Check sheet for the drawn part. Datum: minimum x, y, z corner. Units: mm. A direction names the side the tool comes from. Round coordinates to 2 decimals unless told otherwise and drop trailing zeros. Write each loop counter-clockwise with the first axis right and the second up, starting at its lowest first coordinate (ties: lowest second). Pieces come first, ordered by that corner, then holes. Notation, with made-up numbers: M 55.25,39 L 110.25,39 A30 ccw 110.25,77 Z; hole C 36.5,-23 d4. An arc over 180 degrees is marked long. Put each result on its own line as item: value.
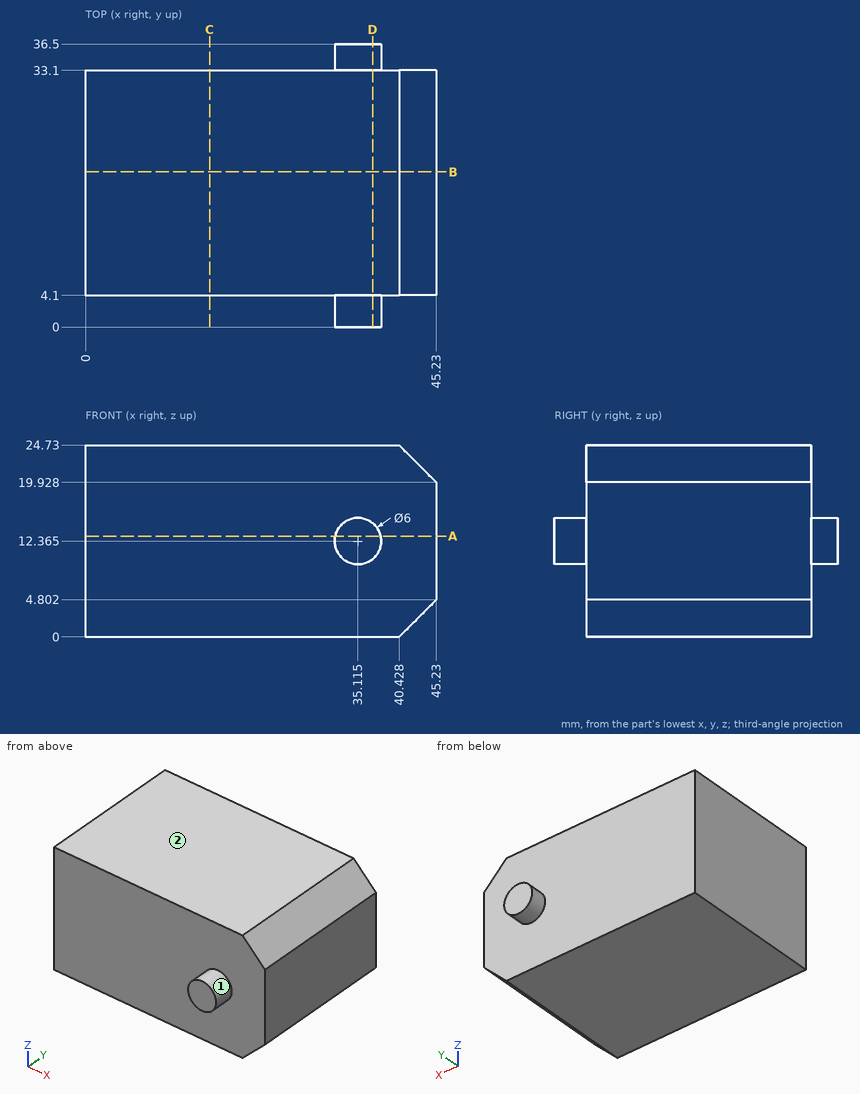
1. Depth check by flat-ended pin: pin 1 Ø1 at (y, z) = (28, 2.5) entering from +X; pin 2 Ø3 at (x, z) = (26.5, 2.5) entering from +Y. Enter the tip coordinate at first touch or a pass-through.
Computed values:
pin 1: stops at x = 43.43
pin 2: stops at y = 33.1
2. Cross-section at D-D (x = 37). Enter the section's corners in (y, z), then the cut area to 3 significant figures.
Computed values:
outline: M 0,10.03 L 4.1,10.03 L 4.1,0 L 33.1,0 L 33.1,10.03 L 36.5,10.03 L 36.5,14.7 L 33.1,14.7 L 33.1,24.73 L 4.1,24.73 L 4.1,14.7 L 0,14.7 Z
area: 752 mm2
3. Cross-section at A-A (z = 13). Enter the section's corners in (x, y).
Computed values:
outline: M 0,4.1 L 32.18,4.1 L 32.18,0 L 38.05,0 L 38.05,4.1 L 45.23,4.1 L 45.23,33.1 L 38.05,33.1 L 38.05,36.5 L 32.18,36.5 L 32.18,33.1 L 0,33.1 Z
4. Cross-section at B-B (y = 20). Enter the section's corners in (x, z).
Computed values:
outline: M 0,0 L 40.43,0 L 45.23,4.8 L 45.23,19.93 L 40.43,24.73 L 0,24.73 Z
5. Cross-section at C-C (x = 16). Enter the section's corners in (y, z), then the cut area to 3 significant figures.
Computed values:
outline: M 4.1,0 L 33.1,0 L 33.1,24.73 L 4.1,24.73 Z
area: 717 mm2
6. Scan lines: probe 1 along Y at (x, z) = (27, 20.5); probe 2 along X at (y, z) = (14.5, 23.5); probe 3 along Z at (x, y) = (43, 8.5). Record each from-to range of solid material in increasing order.
Computed values:
probe 1: y = 4.1 to 33.1
probe 2: x = 0 to 41.66
probe 3: z = 2.57 to 22.16
7. Access from +Z, -Z, +X, -X, +Y, -Y to the whole of each face (thin tool, end or side, straight path). Record for the marked faces 1 and 2.
Computed values:
face 1: -Y
face 2: +Z, +X, -X, +Y, -Y
